Could you check a few things on this model? Use its own coordinates, in mm. Face numbers are marked on the shaded views. A direction names the side the tool comes from. Round coordinates to 2 decimals unless told otherwise and drop trailing zeros. Loops run counter-clockwise (first coordinate to the right, second up) from the corner with the lowest first, then second, coordinate; pieces in that order, holes last.
from build123d import *

# Parameters (mm, degrees)
SKETCH8_W           = 135
SKETCH8_H           = 60
SKETCH8_W_2         = 125
SKETCH8_H_2         = 50
BOSS_EXTRUDE1_DEPTH = 25
SKETCH9_W           = 60
SKETCH9_H           = 5
BOSS_EXTRUDE2_DEPTH = 135


with BuildPart() as part:
    # Sketch8 → Boss-Extrude1 (new, symmetric)
    with BuildSketch(Plane(origin=(0, 0, 0), x_dir=(1, 0, 0), z_dir=(0, 1, 0))):
        Rectangle(SKETCH8_W, SKETCH8_H)
        Rectangle(SKETCH8_W_2, SKETCH8_H_2, mode=Mode.SUBTRACT)
    extrude(amount=BOSS_EXTRUDE1_DEPTH, both=True)

    # Sketch9 → Boss-Extrude2 (add)
    with BuildSketch(Plane.ZY.offset(67.5)):
        with Locations((0, -27.5)):
            Rectangle(SKETCH9_W, SKETCH9_H)
    extrude(amount=-BOSS_EXTRUDE2_DEPTH)


solid = part.part
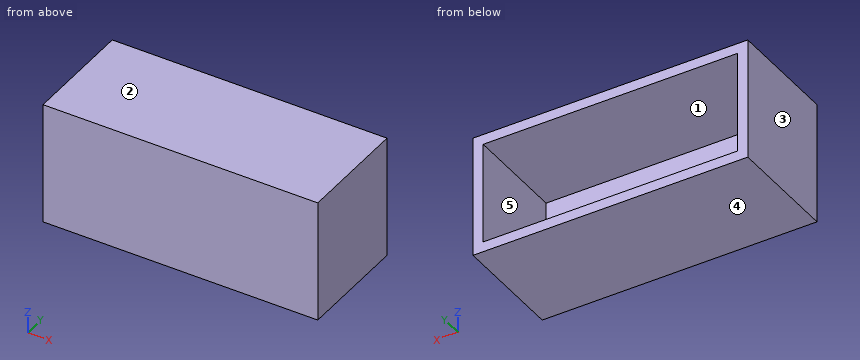
Item 1: If we section it at C-C, the plane x = 53: Please give me the cut outline in (y, z).
Results list:
outline: (-30, -30) - (25, -30) - (25, -25) - (-25, -25) - (-25, 25) - (25, 25) - (25, 30) - (-30, 30) - close
Item 2: If we section it at B-B, the plane z = -15: Please give me the cut outline in (x, y).
Results list:
outline: (-67.5, -30) - (67.5, -30) - (67.5, 25) - (62.5, 25) - (62.5, -25) - (-62.5, -25) - (-62.5, 25) - (-67.5, 25) - close
Item 3: For the marked faces 4 and 5, which set-ups out of +Z, -Z, +X, -X, +Y, -Y let a thin tool reach every point of the face, with its end or its side?
Results list:
face 4: -Z, +X, -X, +Y, -Y
face 5: +Y
Item 4: If I drill on line 1 along X through (y, z) = (22.5, 22.5); line 2 along Z through (x, y) = (20, -10); line 3 along Y through (x, z) = (13, 5.5), over which ranges is the centre line in solid material (lowest first)?
Results list:
line 1: x = -67.5 to -62.5, 62.5 to 67.5
line 2: z = -30 to -25, 25 to 30
line 3: y = -30 to -25
Item 5: If we section it at A-A, the plane y = -21: Please give me the cut outline in (x, z).
Results list:
outline: (-67.5, -30) - (67.5, -30) - (67.5, 30) - (-67.5, 30) - close; hole (-62.5, -25) - (62.5, -25) - (62.5, 25) - (-62.5, 25) - close
Item 6: We'd pull the mould along X, two halves only. Please class the marked faces 1, 2 and 3: released by +X, released by -X, zero draft, split by the parting line, or undercut.
Results list:
face 1: undercut
face 2: zero draft
face 3: released by -X
Item 7: Will this pin go through, and if not, where does the flat tip stop? pin 1 (1.5 mm diameter, centred on x = -8, z = -5.5, fed in from +Y).
Results list:
pin 1: stops at y = -25
